from build123d import *

# Parameters (mm, degrees)
BOSS_EXTRUDE1_DEPTH       = 25
SKETCH2_R                 = 11.2
CUT_EXTRUDE1_DEPTH        = 90.582364336
CHAMFER2_SIZE             = 2
SKETCH11_R                = 11.4
SKETCH11_R_2              = 9
BOSS_EXTRUDE3_DEPTH       = 18
M5_CLEARANCE_HOLE1_D      = 5.5
M5_CLEARANCE_HOLE2_D      = 5.5
M5_CLEARANCE_HOLE2_DEPTH  = 15
F_6_0MM_DOWEL_HOLE1_D     = 6
F_6_0MM_DOWEL_HOLE1_DEPTH = 40
F_6_0MM_DOWEL_HOLE1_TIP   = 1.802581857


with BuildPart() as part:
    # Sketch1 → Boss-Extrude1 (new body)
    with BuildSketch(Plane.XY):
        with BuildLine():
            Line((50, 0), (50, 10))
            Line((50, 10), (35, 10))
            Line((35, 10), (20, 10))
            Line((20, 10), (20, 55))
            Line((20, 55), (35, 55))
            Line((35, 55), (35, 70))
            Line((35, 70), (20, 70))
            Line((20, 70), (3, 57.25))
            ThreePointArc((3, 57.25), (0, 56.25), (-3, 57.25))
            Line((-3, 57.25), (-20, 70))
            Line((-20, 70), (-35, 70))
            Line((-35, 70), (-35, 10))
            Line((-35, 10), (-50, 10))
            Line((-50, 10), (-50, 0))
            Line((-50, 0), (-7.7, 0))
            Line((-7.7, 0), (-7.7, 15))
            ThreePointArc((-7.7, 15), (-7.114213562, 16.414213562), (-5.7, 17))
            Line((-5.7, 17), (5.7, 17))
            ThreePointArc((5.7, 17), (7.114213562, 16.414213562), (7.7, 15))
            Line((7.7, 15), (7.7, 0))
            Line((7.7, 0), (50, 0))
        make_face()
    extrude(amount=BOSS_EXTRUDE1_DEPTH)

    # Sketch2 → Cut-Extrude1 (cut, through all)
    with BuildSketch(Plane(origin=(0, 0, 0), x_dir=(-1, 0, 0), z_dir=(0, 0, -1))):
        with Locations((0, 37)):
            Circle(SKETCH2_R)
    extrude(amount=-CUT_EXTRUDE1_DEPTH, mode=Mode.SUBTRACT)

    # Chamfer2
    chamfer2_edges = [part.edges().sort_by_distance(p)[0] for p in [
        (-35, 70, 12.5),
        (35, 70, 12.5),
        (35, 55, 12.5),
        (20, 55, 12.5),
    ]]
    chamfer(chamfer2_edges, length=CHAMFER2_SIZE)

    # Sketch11 → Boss-Extrude3 (add)
    with BuildSketch(Plane.XY.offset(25)):
        with Locations((0, 37)):
            Circle(SKETCH11_R)
        with Locations((0, 37)):
            Circle(SKETCH11_R_2, mode=Mode.SUBTRACT)
    extrude(amount=-BOSS_EXTRUDE3_DEPTH)

    # M5 Clearance Hole1 (through all)
    with Locations(Plane(origin=(0, 10, 0), x_dir=(1, 0, 0), z_dir=(0, 1, 0))):
        with Locations((42.5, -18.5), (42.5, -6.5), (-42.5, -18.5), (-42.5, -6.5)):
            Hole(M5_CLEARANCE_HOLE1_D / 2)

    # M5 Clearance Hole2
    with Locations(Plane(origin=(0, 70, 0), x_dir=(1, 0, 0), z_dir=(0, 1, 0))):
        with Locations((28.5, -12.5)):
            Hole(M5_CLEARANCE_HOLE2_D / 2, depth=M5_CLEARANCE_HOLE2_DEPTH)

    # Ø6.0mm Dowel Hole1
    with Locations(Plane(origin=(0, 70, 0), x_dir=(1, 0, 0), z_dir=(0, 1, 0))):
        with Locations((-29, -12.5)):
            Hole(F_6_0MM_DOWEL_HOLE1_D / 2, depth=F_6_0MM_DOWEL_HOLE1_DEPTH)
            with Locations((0, 0, -(F_6_0MM_DOWEL_HOLE1_DEPTH + F_6_0MM_DOWEL_HOLE1_TIP / 2))):  # 118° drill point
                Cone(0, F_6_0MM_DOWEL_HOLE1_D / 2, F_6_0MM_DOWEL_HOLE1_TIP, mode=Mode.SUBTRACT)


solid = part.part
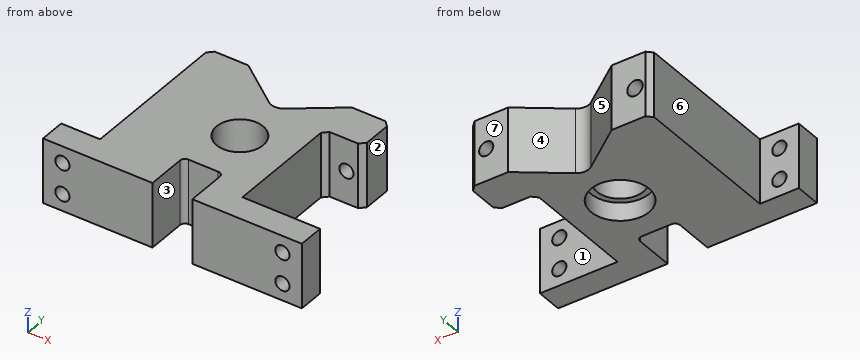
CAD build for the part. Positions are in the model's coordinates, mm. Face numbers are marked on the shaded views. A direction names the side the tool comes from. Round coordinates to 2 decimals unless told otherwise and drop trailing zeros. Write each loop counter-clockwise with the first axis right and the second up, starting at its lowest first coordinate (ties: lowest second). Pieces come first, ordered by that corner, then holes. Notation, with made-up numbers: M -13.75,11 L 10.25,11 A31 cw 10.25,39 Z; hole C -24,-38 d8. An arc over 180 degrees is marked long. Put each result on its own line as item: value. Start each with the question number.
1) Saw through at B-B, the plane z = 18.5. Count the separate pieces of the cut face and the enclosed holes in it, and give its area (3 significant figures).
2) Saw through at C-C, the plane x = -42.5. Write the cut outline in (y, z), and give its area (3 significant figures).
3) 3-axis set-ups, long thin cutter, end or side, ignore diameter. For the marked faces 1, 2 and 3: which of +Z, -Z, +X, -X, +Y, -Y reach the whole face in a straight line?
4) Saw through at A-A, the plane y = 37. Write the cut outline in (x, z), and give its area (3 significant figures).
5) Drill centre lines: probe 1 along X at (y, z) = (7.75, 18.5); probe 2 along Y at (x, z) = (0, 2); probe 3 along Z at (x, y) = (-42.5, 5.75). Where is each one in solid material? Low to high. Write a range as [from, to].
6) Pin check, flat tips, straight feed: pin 1 Ø23.5 at (x, y) = (0, 37) entering from +Z; pin 2 Ø5 at (x, z) = (-29, 12.5) entering from +Y; pin 3 Ø4.5 at (x, z) = (-40, 11) entering from +Y; pin 4 Ø2 at (y, z) = (12.5, 16) entering from +X. Stop position of each tip, or through.
7) Saw through at D-D, the plane y = 13.5. Write the cut outline in (x, z), and give its area (3 significant figures).
8) Pull direction X, two halves, no side cores. Call the marked faces 4, 5, 6 and 7: pulls with the +X half, pulls with the -X half, needs draft (parallel to the pull), parting line crosses it, or undercut.
Resolved:
1. separate pieces: 3
1. enclosed holes: 1
1. area: 3,600 mm²
2. outline: M 0,0 L 10,0 L 10,3.75 L 0,3.75 Z; M 0,9.25 L 10,9.25 L 10,15.75 L 0,15.75 Z; M 0,21.25 L 10,21.25 L 10,25 L 0,25 Z
2. area: 140 mm²
3. face 1: +Z, -Z, +X
3. face 2: +Z, -Z, +X, +Y
3. face 3: +Z, -Z, -Y
4. outline: M -35,0 L -11.2,0 L -11.2,7 L -9,7 L -9,25 L -35,25 Z; M 9,7 L 11.2,7 L 11.2,0 L 20,0 L 20,25 L 9,25 Z; hole C -29,12.5 d6
4. area: 866 mm²
5. probe 1: [-50, -45.25], [-39.75, -7.7], [7.7, 39.75], [45.25, 50]
5. probe 2: [17, 25.8], [48.2, 56.25]
5. probe 3: [0, 3.75], [9.25, 15.75], [21.25, 25]
6. pin 1: z = 25
6. pin 2: y = 29.7
6. pin 3: y = 10
6. pin 4: x = 20
7. outline: M -35,0 L -7.7,0 L -7.7,25 L -35,25 Z; M 7.7,0 L 20,0 L 20,25 L 7.7,25 Z
7. area: 990 mm²
8. face 4: undercut
8. face 5: undercut
8. face 6: pulls with the -X half
8. face 7: needs draft
